from build123d import *

# Parameters (mm, degrees)
REVOLVE1_ANGLE       = 70
BOSS_EXTRUDE1_START  = -17.5895
BOSS_EXTRUDE1_DEPTH  = 17.5895
BOSS_EXTRUDE2_DEPTH  = 3.175
BOSS_EXTRUDE3_DEPTH  = 12.7
CUT_SWEEP1_PROFILE_R = 3.302
CUT_EXTRUDE7_DEPTH   = 27.94
BOSS_EXTRUDE4_REACH  = 54.438
CUT_EXTRUDE8_DEPTH   = 1.7145
CUT_EXTRUDE9_DEPTH   = 54.83153704
BOSS_EXTRUDE5_REACH  = 52.224
SKETCH45_R           = 5
SKETCH45_R_2         = 3.302


with BuildPart() as part:
    # Sketch3 → Revolve1 (revolve, symmetric)
    with BuildSketch(Plane.XY) as revolve1_sk:
        Polygon((-44.1325, 4.03225), (-23.8125, 4.03225), (-23.8125, -13.55725), (-44.1325, -13.55725), (-44.1325, -0.85725), (-30.7975, -0.85725), (-30.7975, 0.85725), (-44.1325, 0.85725), align=None)
    revolve(axis=Axis((0, -1086.549659172, 0), (0, 1, 0)), revolution_arc=REVOLVE1_ANGLE / 2)
    revolve(revolve1_sk.sketch, axis=Axis((0, -1086.549659172, 0), (0, -1, 0)), revolution_arc=REVOLVE1_ANGLE / 2)

    # Sketch10 → Boss-Extrude1 (add)
    with BuildSketch(Plane(origin=(0, 4.03225, 0), x_dir=(1, 0, 0), z_dir=(0, 1, 0)).offset(BOSS_EXTRUDE1_START)):
        with BuildLine():
            Line((-19.506058055, 13.658288891), (-19.506058055, -13.658288891))
            ThreePointArc((-19.506058055, -13.658288891), (-23.8125, 0), (-19.506058055, 13.658288891))
        make_face()
    extrude(amount=BOSS_EXTRUDE1_DEPTH)

    # Sketch11 → Boss-Extrude2 (add)
    with BuildSketch(Plane(origin=(0, 4.03225, 0), x_dir=(1, 0, 0), z_dir=(0, 1, 0))):
        Polygon((-36.151227595, 25.313362077), (-19.506058055, 25.313362077), (-19.506058055, 13.658288891), align=None)
        Polygon((-36.151227595, -25.313362077), (-19.506058055, -25.313362077), (-19.506058055, -13.658288891), align=None)
    extrude(amount=-BOSS_EXTRUDE2_DEPTH)

    # Sketch12 → Boss-Extrude3 (add)
    with BuildSketch(Plane.XZ.offset(13.55725)):
        Polygon((-36.151227595, 25.313362077), (-19.506058055, 25.313362077), (-19.506058055, 13.658288891), align=None)
        Polygon((-36.151227595, -25.313362077), (-19.506058055, -13.658288891), (-19.506058055, -25.313362077), align=None)
    extrude(amount=-BOSS_EXTRUDE3_DEPTH)

    # Cut-Sweep1: sweep along a path in Sketch14
    with BuildLine(Plane(origin=(0, -6.95325, 0), x_dir=(-1, 0, 0), z_dir=(0, -1, 0))) as cut_sweep1_path:
        Line((9.675589129, 4.493239256), (40.02699074, 18.588102876))
    # Cut-Sweep1 profile (on start of the path) → Cut-Sweep1 (sweep, cut)
    with BuildSketch(Plane(origin=(-9.675589129, -6.95325, -4.493239256), x_dir=(0.421188531725906, 0, -0.9069731091617742), z_dir=(-0.9069731091617742, -3.1111435997184875e-15, -0.421188531725906))):
        Circle(CUT_SWEEP1_PROFILE_R)
    cut_sweep1 = sweep(path=cut_sweep1_path.line, mode=Mode.SUBTRACT)

    # Mirror1: Cut-Sweep1 across plane
    add(cut_sweep1.mirror(Plane.XY), mode=Mode.SUBTRACT)

    # Sketch37 → Cut-Extrude7 (cut)
    with BuildSketch(Plane(origin=(0, 0, 0), x_dir=(-0.42118853172590587, -1.4445522614505264e-15, 0.9069731091617743), z_dir=(-0.9069731091617742, -3.103462646485123e-15, -0.4211885317259058))):
        Polygon((-5.0165, -4.056972375), (-5.0165, -9.849527625), (0, -12.745805251), (5.0165, -9.849527625), (5.0165, -4.056972375), (0, -1.160694749), align=None)
    cut_extrude7 = extrude(amount=CUT_EXTRUDE7_DEPTH, mode=Mode.SUBTRACT)

    # Mirror2: Cut-Extrude7 across plane
    add(cut_extrude7.mirror(Plane.XY), mode=Mode.SUBTRACT)

    # Sketch38 → Boss-Extrude4 (add, up to next)
    with BuildSketch(Plane(origin=(0, -0.85725, 0), x_dir=(1, 0, 0), z_dir=(0, 1, 0)), mode=Mode.PRIVATE) as boss_extrude4_sk1:
        Polygon((-25.227835084, 17.664720299), (-19.506058055, 17.664720299), (-19.506058055, 13.658288891), align=None)
    boss_extrude4_tool1 = extrude(boss_extrude4_sk1.sketch, amount=BOSS_EXTRUDE4_REACH, mode=Mode.PRIVATE) - part.part
    # Sketch38 → Boss-Extrude4 (add, up to next)
    with BuildSketch(Plane(origin=(0, -0.85725, 0), x_dir=(1, 0, 0), z_dir=(0, 1, 0)), mode=Mode.PRIVATE) as boss_extrude4_sk2:
        Polygon((-25.227835084, -17.664720299), (-19.506058055, -13.658288891), (-19.506058055, -17.664720299), align=None)
    boss_extrude4_tool2 = extrude(boss_extrude4_sk2.sketch, amount=BOSS_EXTRUDE4_REACH, mode=Mode.PRIVATE) - part.part
    add(boss_extrude4_tool1.solids().sort_by_distance((-21.413317, -0.85725, -16.329243))[0])
    add(boss_extrude4_tool2.solids().sort_by_distance((-21.413317, -0.85725, 16.329243))[0])

    # Sketch39 → Cut-Extrude8 (cut)
    with BuildSketch(Plane.XZ.offset(-0.85725)):
        with BuildLine():
            Line((-25.227835084, -17.664720299), (-25.227835084, 17.664720299))
            ThreePointArc((-25.227835084, 17.664720299), (-30.7975, 0), (-25.227835084, -17.664720299))
        make_face()
    extrude(amount=CUT_EXTRUDE8_DEPTH, mode=Mode.SUBTRACT)

    # Sketch44 → Cut-Extrude9 (cut, through all)
    with BuildSketch(Plane.XZ.offset(13.55725)):
        with BuildLine():
            Line((-36.151227595, 25.313362077), (-36.151227595, -25.313362077))
            ThreePointArc((-36.151227595, -25.313362077), (-44.1325, 0), (-36.151227595, 25.313362077))
        make_face()
    extrude(amount=-CUT_EXTRUDE9_DEPTH, mode=Mode.SUBTRACT)

    # Boss-Extrude5: up to this plane
    boss_extrude5_end = Plane(origin=(-36.151227595, 4.03225, 25.313362077), z_dir=(1, 0, 0))
    # Sketch45 → Boss-Extrude5 (add, up to the surface)
    with BuildSketch(Plane(origin=(-39.906816803, 0, -18.532295396), x_dir=(-0.42118853172590587, -1.4445522614505264e-15, 0.9069731091617743), z_dir=(-0.9069731091617742, -3.103462646485123e-15, -0.4211885317259058)), mode=Mode.PRIVATE) as boss_extrude5_sk1:
        with Locations((0, -6.95325)):
            Circle(SKETCH45_R)
        with Locations((0, -6.95325)):
            Circle(SKETCH45_R_2, mode=Mode.SUBTRACT)
    boss_extrude5_tool1 = split(extrude(boss_extrude5_sk1.sketch, amount=-BOSS_EXTRUDE5_REACH, mode=Mode.PRIVATE), bisect_by=boss_extrude5_end, keep=Keep.BOTH, mode=Mode.PRIVATE)
    boss_extrude5 = boss_extrude5_tool1.solids().sort_by_distance((-37.860439, -6.95325, -22.938896))[0]
    add(boss_extrude5)

    # Mirror3: Boss-Extrude5 across plane
    add(boss_extrude5.mirror(Plane.XY))


solid = part.part
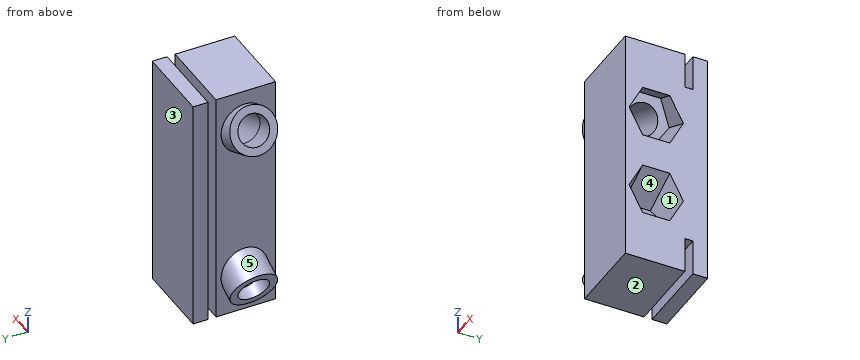
Build history of the part. All positions in model axes, mm. Face numbers are marked on the shaded views. A direction names the side the tool comes from. Round coordinates to 2 decimals unless told otherwise and drop trailing zeros. Loops run counter-clockwise (first coordinate to the right, second up) from the corner with the lowest first, then second, coordinate; pieces in that order, holes last. Notation, with made-up numbers: (-31, 60.25) -> (20, 60.25) arc R19 ccw to (20, 78.25) -> close; hole circle Ø9 at (52.25, 0.5). An arc over 180 degrees is marked (long way). Answer in a Markdown table with one row per item.
Item 1: Pin check, flat tips, straight feed: pin 1 (1.4 mm diameter, centred on y = 0, z = -1.5, fed in from -X); pin 2 (6.5 mm diameter, centred on y = -4, z = 5.5, fed in from -X); pin 3 (1 mm diameter, centred on x = -38, y = -4.5, fed in from +Z). Stop position of each tip, or through.
Answers below:
| item | result |
|---|---|
| pin 1 | stops at x = -25.23 |
| pin 2 | stops at x = -36.15 |
| pin 3 | stops at z = 22.71 |
Item 2: Saw through at C-C (x = -35). State how many separate pieces and enclosed holes the cut face has, and give its area (3 significant figures).
Answers below:
| item | result |
|---|---|
| separate pieces | 2 |
| enclosed holes | 2 |
| area | 728 mm² |
Item 3: Mould opens along Z. For the marked faces 1, 2 and 3 say: +Z half, -Z half, draft (parallel to the pull), parting line (faces both ways), or undercut.
Answers below:
| item | result |
|---|---|
| face 1 | undercut |
| face 2 | -Z half |
| face 3 | draft |
Item 4: Which spindle directions (+Z, -Z, +X, -X, +Y, -Y) get a long thin tool onto all of the face, cutting with end or side? Do the marked faces 4 and 5. Say none if no direction does.
Answers below:
| item | result |
|---|---|
| face 4 | +X |
| face 5 | none |
Item 5: Saw through at B-B (y = -4.75). Write the cut outline in (x, z).
Answers below:
| item | result |
|---|---|
| outline | (-41.8, -14.46) -> (-40.94, -16.3) -> (-26.38, -9.54) -> (-27.45, -7.22) -> (-19.51, -3.53) -> (-19.51, 3.53) -> (-27.45, 7.22) -> (-26.38, 9.54) -> (-40.94, 16.3) -> (-41.8, 14.46) -> (-36.15, 11.84) -> (-36.15, -11.84) -> close; (-38.87, -20.76) -> (-38.02, -22.6) -> (-36.15, -21.74) -> (-36.15, -25.31) -> (-19.51, -25.31) -> (-19.51, -14.59) -> (-23.23, -16.32) -> (-24.3, -14) -> close; (-38.87, 20.76) -> (-24.3, 14) -> (-23.23, 16.32) -> (-19.51, 14.59) -> (-19.51, 25.31) -> (-36.15, 25.31) -> (-36.15, 21.74) -> (-38.02, 22.6) -> close |
Item 6: Saw through at D-D (y = -11). Write the cut outline in (x, z).
Answers below:
| item | result |
|---|---|
| outline | (-41.14, -15.87) -> (-38.67, -21.2) -> (-36.15, -20.03) -> (-36.15, -25.31) -> (-19.51, -25.31) -> (-19.51, -12.39) -> (-24.07, -14.51) -> (-26.61, -9.03) -> (-19.51, -5.72) -> (-19.51, 5.72) -> (-26.61, 9.03) -> (-24.07, 14.51) -> (-19.51, 12.39) -> (-19.51, 25.31) -> (-36.15, 25.31) -> (-36.15, 20.03) -> (-38.67, 21.2) -> (-41.14, 15.87) -> (-36.15, 13.55) -> (-36.15, -13.55) -> close |
Item 7: Drill centre lines: L1, parallel to Y at x = -31.5, z = 7; L2, parallel to Z at x = -35.25, y = -4.75; L3, parallel to Z at x = -35.75, y = -9.5. Where is each one in solid material? Low to high. Write a range as [from, to].
Answers below:
| item | result |
|---|---|
| L1 | y = [-13.56, -0.86], [0.86, 4.03] |
| L2 | z = [-25.31, -19.08], [-13.66, 13.66], [19.08, 25.31] |
| L3 | z = [-25.31, -18.92], [-14.28, 14.28], [18.92, 25.31] |
Item 8: Saw through at A-A (z = -0.5). Write the cut outline in (x, y).
Answers below:
| item | result |
|---|---|
| outline | (-36.15, -13.56) -> (-19.51, -13.56) -> (-19.51, 4.03) -> (-36.15, 4.03) -> (-36.15, 0.86) -> (-25.23, 0.86) -> (-25.23, -0.86) -> (-36.15, -0.86) -> close |
